Verification items for the finished model (mm, model axes). Face numbers are marked on the shaded views. A direction names the side the tool comes from. Coordinates: 2 decimals unless noted, no trailing zeros. Order: outer loops, then holes, each group sorted by start corner. A loop starts at its lowest first (then second) coordinate and runs counter-clockwise, first axis right, second up. Notation, with made-up numbers: M 29,29.25 L 46,29.25 A13 cw 46,52.25 Z; hole C -35,37 d2. An arc over 180 degrees is marked long. Return JSON: item names as keys, results as strings. Group by question number.
Q1. Section check B-B, the plane z = 19.5. Enter the section's corners in (x, y).
Q2. Access from +Z, -Z, +X, -X, +Y, -Y to the whole of each face (thin tool, end or side, straight path). Record for the marked faces 1, 2, 3, 4 and 5.
Q3. Thickness scan on probe 1 along Y at (x, z) = (-9, 20.55); probe 2 along X at (y, z) = (-1.5, 18.75); probe 3 along Z at (x, y) = (12.75, -47). Record the ranges inside material, lowest first.
Q4. Section check D-D, the plane x = 3.25. Enter the section's corners in (y, z) (3 decimals).
Q5. Section check C-C, the plane y = -29. Enter the section's corners in (x, z).
Q6. Go/stop test with flat-tipped pins: pin 1 Ø12 at (y, z) = (-29, 13) entering from +X; pin 2 Ø5 at (x, y) = (9, 0) entering from +Z; pin 3 Ø8 at (x, y) = (9, -47.18) entering from +Z; pin 4 Ø2 at (x, z) = (-10, 3) entering from -Y. Record where each tip stops, or that it passes through.
Q7. Section check A-A, the plane x = -9. Enter the section's corners in (y, z).
from build123d import *

# Parameters (mm, degrees)
ESBO_O1_R                = 1.598160281
ESBO_O1_R_2              = 1.600993429
RESSALTO_EXTRUS_O1_DEPTH = 5
ESBO_O2_W                = 8.00000038
ESBO_O2_H                = 11.528000702
RESSALTO_EXTRUS_O2_DEPTH = 17.480363
ESBO_O3_W                = 8.00000038
ESBO_O3_H                = 4
RESSALTO_EXTRUS_O3_DEPTH = 44.418848
ESBO_O4_W                = 4
ESBO_O4_H                = 6.000686184
RESSALTO_EXTRUS_O4_DEPTH = 10
ESBO_O5_W                = 4
ESBO_O5_H                = 6
RESSALTO_EXTRUS_O5_DEPTH = 10
FILETE1_R                = 10
FILETE2_R                = 10
ESBO_O6_R                = 2.5
CORTE_EXTRUS_O1_DEPTH    = 10


with BuildPart() as part:
    # Esboço1 → Ressalto-extrusão1 (new body)
    with BuildSketch(Plane.XY):
        with BuildLine():
            Line((-10.199065979, -3.817665654), (-4.00000019, -5.764999893))
            Line((-4.00000019, -5.764999893), (4.00000019, -5.764999893))
            Line((4.00000019, -5.764999893), (10.197782, -3.817301838))
            ThreePointArc((10.197782, -3.817301838), (12.999977706, 0.001566069), (10.195969576, 3.8191034))
            Line((10.195969576, 3.8191034), (4.00000019, 5.763000809))
            Line((4.00000019, 5.763000809), (-4.00000019, 5.763000809))
            Line((-4.00000019, 5.763000809), (-10.199143851, 3.815503142))
            ThreePointArc((-10.199143851, 3.815503142), (-13.000622723, -0.001109837), (-10.199065979, -3.817665654))
        make_face()
        with Locations((8.997973452, 0.000616233)):
            Circle(ESBO_O1_R, mode=Mode.SUBTRACT)
        with Locations((-9.000145119, -0.001069025)):
            Circle(ESBO_O1_R_2, mode=Mode.SUBTRACT)
    extrude(amount=RESSALTO_EXTRUS_O1_DEPTH)

    # Esboço2 → Ressalto-extrusão2 (add)
    with BuildSketch(Plane.XY.offset(5)):
        with Locations((0, -0.000999542)):
            Rectangle(ESBO_O2_W, ESBO_O2_H)
    extrude(amount=RESSALTO_EXTRUS_O2_DEPTH)

    # Esboço3 → Ressalto-extrusão3 (add)
    with BuildSketch(Plane.XZ.offset(5.764999893)):
        with Locations((0, 20.480363203)):
            Rectangle(ESBO_O3_W, ESBO_O3_H)
    extrude(amount=RESSALTO_EXTRUS_O3_DEPTH)

    # Esboço4 → Ressalto-extrusão4 (add)
    with BuildSketch(Plane.ZY.offset(4.00000019)):
        with Locations((20.480363203, -47.183504361)):
            Rectangle(ESBO_O4_W, ESBO_O4_H)
    extrude(amount=RESSALTO_EXTRUS_O4_DEPTH)

    # Esboço5 → Ressalto-extrusão5 (add)
    with BuildSketch(Plane(origin=(4.00000019, 0, 0), x_dir=(0, 0, -1), z_dir=(1, 0, 0))):
        with Locations((-20.480363203, -47.183847453)):
            Rectangle(ESBO_O5_W, ESBO_O5_H)
    extrude(amount=RESSALTO_EXTRUS_O5_DEPTH)

    # Filete1
    filete1_edges = [part.edges().sort_by_distance(p)[0] for p in [
        (0, -5.764999893, 18.480363203),
    ]]
    fillet(filete1_edges, radius=FILETE1_R)

    # Filete2
    filete2_edges = [part.edges().sort_by_distance(p)[0] for p in [
        (0, 5.763000809, 22.480363),
    ]]
    fillet(filete2_edges, radius=FILETE2_R)

    # Esboço6 → Corte-extrusão1 (cut)
    with BuildSketch(Plane(origin=(0, 0, 18.480363203), x_dir=(-1, 0, 0), z_dir=(0, 0, -1))):
        with Locations((-9.00000019, -47.183786187)):
            Circle(ESBO_O6_R)
        with Locations((9.00000019, -47.183565627)):
            Circle(ESBO_O6_R)
    extrude(amount=-CORTE_EXTRUS_O1_DEPTH, mode=Mode.SUBTRACT)


solid = part.part
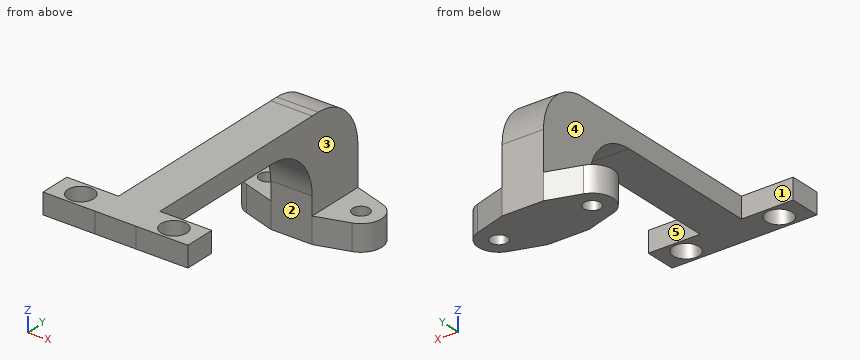
Numbers:
{
 "1": {"outline": "M -14,-50.18 L 14,-50.18 L 14,-44.18 L 4,-44.18 L 4,2.89 L -4,2.89 L -4,-44.18 L -14,-44.18 Z; hole C -9,-47.18 d5; hole C 9,-47.18 d5"},
 "2": {"face 1": "+Z, -Z, -X, +Y", "face 2": "-Z, +X, -X, -Y", "face 3": "+Z, +X, +Y", "face 4": "+Z, -X, +Y", "face 5": "+Z, -Z, +X, +Y"},
 "3": {"probe 1": "y = -50.18 to -49.68, -44.68 to -44.18", "probe 2": "x = -4 to 4", "probe 3": "z = 18.48 to 22.48"},
 "4": {"outline": "M -50.184,18.48 L -15.765,18.48 A10 cw -5.765,8.48 L -5.765,0 L 5.763,0 L 5.763,12.48 A10 ccw -4.237,22.48 L -50.184,22.48 Z"},
 "5": {"outline": "M -4,18.48 L 4,18.48 L 4,22.48 L -4,22.48 Z"},
 "6": {"pin 1": "stops at x = 4", "pin 2": "stops at z = 5", "pin 3": "stops at z = 22.48", "pin 4": "stops at y = -4.19"},
 "7": {"outline": "M -50.18,18.48 L -49.68,18.48 L -49.68,22.48 L -50.18,22.48 Z; M -44.68,18.48 L -44.18,18.48 L -44.18,22.48 L -44.68,22.48 Z; M -4.19,0 L -1.6,0 L -1.6,5 L -4.19,5 Z; M 1.6,0 L 4.19,0 L 4.19,5 L 1.6,5 Z"}
}
